```python
from build123d import *

# Parameters (mm, degrees)
F2_W      = 14
F2_H      = 14
F2_R      = 5
F3_DEPTH  = 14
F4_ANGLE  = -90
F6_R      = 1
F8_DEPTH  = 14.001
F7_R      = 1
F9_DEPTH  = 2.1020206144
F10_SIZE2 = 1.5
F10_SIZE  = 1.5


with BuildPart() as f3:
    # F2 (on Front) → F3 (new body)
    with BuildSketch(Plane.XZ):
        Rectangle(F2_W, F2_H)
        Circle(F2_R, mode=Mode.SUBTRACT)
    extrude(amount=F3_DEPTH)


with BuildPart() as f4_1:
    # F4: copy of F3
    add(f3.part.rotate(Axis((7, 0, 0), (0, 0, -1)), F4_ANGLE))


with BuildPart() as f3_1:
    add(f3.part)

    # F5: union F4_1
    add(f4_1.part)

    # F6 (on face) → F8 (cut, through all)
    with BuildSketch(Plane(origin=(0, 0, -7), x_dir=(1, 0, 0), z_dir=(0, 0, -1))):
        with Locations((0, 7)):
            Circle(F6_R)
        with Locations((15, 7)):
            Circle(F6_R)
    extrude(amount=-F8_DEPTH, mode=Mode.SUBTRACT)

    # F7 (on face) → F9 (cut, through all)
    with BuildSketch(Plane(origin=(-7, 0, 0), x_dir=(0, -1, 0), z_dir=(-1, 0, 0))):
        with Locations((7, 0)):
            Circle(F7_R)
    extrude(amount=-F9_DEPTH, mode=Mode.SUBTRACT)

    # F10
    f10_edges = [f3_1.edges().sort_by_distance(p)[0] for p in [
        (-1, -7, -7),
        (14, -7, -7),
        (-1, -7, 7),
        (14, -7, 7),
        (-7, -6, 0),
    ]]
    chamfer(f10_edges, length=F10_SIZE, length2=F10_SIZE2)


solid = f3_1.part
```
Check sheet for the modelled part. Datum: model origin and axes. Units: mm. A direction names the side the tool comes from. Coordinates: 2 decimals unless noted, no trailing zeros. Write each loop counter-clockwise with the first axis right and the second up, starting at its lowest first coordinate (ties: lowest second). Pieces come first, ordered by that corner, then holes. Notation, with made-up numbers: (-21, 43) - (33, 43) arc R16 ccw to (33, 55) - close; hole circle Ø4 at (17, 38). An arc over 180 degrees is marked (long way). One line per question, with ' | ' between items.
Item 1: Thickness scan on line 1 (X direction, y = -7, z = -5.2); line 2 (Y direction, x = 15, z = -5); line 3 (Z direction, x = 10.5, y = -7). Record the ranges inside material, lowest first. Write a range as [from, to].
Determined:
line 1: x = [-7, -1], [1, 14], [16, 21] | line 2: y = [-14, -8], [-6, 0] | line 3: z = [-7, -5], [5, 7]
Item 2: Sectioned sample at B-B on x = -3. Record the boundary of the cut face in (y, z).
Determined:
outline: (-14, -7) - (0, -7) - (0, -4) - (-14, -4) - close; (-14, 4) - (0, 4) - (0, 7) - (-14, 7) - close
Item 3: Access from +Z, -Z, +X, -X, +Y, -Y to the whole of each face (thin tool, end or side, straight path). Record for faces 4 (the face through (4.619, -6.902, -1.915)), 5 (the face through (7, -7, 0)), 6 (the face through (-5.204, -7.954, 0.3)).
Determined:
face 4: +Y, -Y | face 5: +X | face 6: -X
Item 4: Sectioned sample at A-A on x = 0. Record the boundary of the cut face in (y, z).
Determined:
outline: (-14, -7) - (-9.5, -7) - (-8, -5.5) - (-8, -5) - (-14, -5) - close; (-14, 5) - (-8, 5) - (-8, 5.5) - (-9.5, 7) - (-14, 7) - close; (-6, -5.5) - (-4.5, -7) - (0, -7) - (0, -5) - (-6, -5) - close; (-6, 5) - (0, 5) - (0, 7) - (-4.5, 7) - (-6, 5.5) - close
Item 5: Sectioned sample at D-D on y = -12.5. Record the boundary of the cut face in (x, z).
Determined:
outline: (-7, -7) - (21, -7) - (21, 7) - (-7, 7) - close; hole circle Ø10 at (0, 0)
Item 6: Gauge pin test, flat ends, axial feed: P1, Ø2.5, axis at x = 0, y = -7, coming from the -Z side; P2, Ø2, axis at x = 4.5, z = -2, coming from the +Y side; P3, Ø2.5, axis at x = 0, y = -7, coming from the +Z side; P4, Ø1.6, axis at y = -7, z = 0, coming from the -X side. Record the tip position at first contact, or that the pin passes through.
Determined:
P1: stops at z = -5.75 | P2: stops at y = 0 | P3: stops at z = 5.75 | P4: stops at x = 4.94
Item 7: Mould release check, pull along Y, two halves, no side actions. Record for faces 1 (the face through (0.954, -7.3, -5.204)), 2 (the face through (10, 0, 0)), 3 (the face through (-7, -10, 0)): pulls with the +Y half, pulls with the -Y half, needs draft (parallel to the pull), parting line crosses it, or undercut.
Determined:
face 1: undercut | face 2: pulls with the +Y half | face 3: needs draft
Item 8: Sectioned sample at C-C on z = 0. Record the boundary of the cut face in (x, y), plus the area to 3 significant figures.
Determined:
outline: (-7, -14) - (-5, -14) - (-5, -8) - (-5.5, -8) - (-7, -9.5) - close; (-7, -4.5) - (-5.5, -6) - (-5, -6) - (-5, 0) - (-7, 0) - close; (5, -14) - (21, -14) - (21, -12) - (7, -12) - (7, -2) - (21, -2) - (21, 0) - (5, 0) - close | area: 106 mm2
